Geometry check sheet. Reference: the model listing, model coordinates, mm. Coordinates: 2 decimals unless noted, no trailing zeros. Write each loop counter-clockwise with the first axis right and the second up, starting at its lowest first coordinate (ties: lowest second). Pieces come first, ordered by that corner, then holes. Notation, with made-up numbers: (-19, -24.75) -> (6, -24.75) arc R25 cw to (6, -7.75) -> close; hole circle Ø9 at (-29.75, 54). An arc over 180 degrees is marked (long way). One line per question, with ' | ' between items.
```python
from build123d import *

# Parameters (mm, degrees)
BOSS_EXTRUDE1_DEPTH = 450
SKETCH2_R           = 3
CUT_EXTRUDE1_DEPTH  = 4.5
SKETCH3_R           = 1.75
CUT_EXTRUDE2_DEPTH  = 451.09610085
LPATTERN1_COUNT     = 6
LPATTERN1_PITCH     = 80


with BuildPart() as part:
    # Sketch1 → Boss-Extrude1 (new body)
    with BuildSketch(Plane.XY):
        with BuildLine():
            Line((6.624531067, 2.444), (6.139791576, 2.444))
            ThreePointArc((6.139791576, 2.444), (5.3, 1.894), (6.139791576, 1.344))
            Line((6.139791576, 1.344), (6.624531067, 1.344))
            ThreePointArc((6.624531067, 1.344), (6.975900024, 0.857004226), (7.5, 0.563841739))
            Line((7.5, 0.563841739), (7.5, -4.2))
            Line((7.5, -4.2), (6.7, -5))
            Line((6.7, -5), (-6.7, -5))
            Line((-6.7, -5), (-7.5, -4.2))
            Line((-7.5, -4.2), (-7.5, 0.563841739))
            ThreePointArc((-7.5, 0.563841739), (-6.975900024, 0.857004226), (-6.624531067, 1.344))
            Line((-6.624531067, 1.344), (-6.139791576, 1.344))
            ThreePointArc((-6.139791576, 1.344), (-5.3, 1.894), (-6.139791576, 2.444))
            Line((-6.139791576, 2.444), (-6.624531067, 2.444))
            ThreePointArc((-6.624531067, 2.444), (-6.975900024, 2.930995774), (-7.5, 3.224158261))
            Line((-7.5, 3.224158261), (-7.5, 4.2))
            Line((-7.5, 4.2), (-6.7, 5))
            Line((-6.7, 5), (6.7, 5))
            Line((6.7, 5), (7.5, 4.2))
            Line((7.5, 4.2), (7.5, 3.224158261))
            ThreePointArc((7.5, 3.224158261), (6.975900024, 2.930995774), (6.624531067, 2.444))
        make_face()
    extrude(amount=-BOSS_EXTRUDE1_DEPTH)

    # Sketch2 → Cut-Extrude1 (cut)
    with BuildSketch(Plane(origin=(0, 5, 0), x_dir=(1, 0, 0), z_dir=(0, 1, 0))):
        with Locations(Location((0, 25, 0), (0, 0, 270))):
            Circle(SKETCH2_R)
    cut_extrude1 = extrude(amount=-CUT_EXTRUDE1_DEPTH, mode=Mode.SUBTRACT)

    # Sketch3 → Cut-Extrude2 (cut, through all)
    with BuildSketch(Plane(origin=(0, 0.5, 0), x_dir=(1, 0, 0), z_dir=(0, 1, 0))):
        with Locations(Location((0, 25, 0), (0, 0, 270))):
            Circle(SKETCH3_R)
    cut_extrude2 = extrude(amount=-CUT_EXTRUDE2_DEPTH, mode=Mode.SUBTRACT)

    # LPattern1: Cut-Extrude1, Cut-Extrude2 ×6
    with Locations(*[(0, 0, -i * LPATTERN1_PITCH) for i in range(1, LPATTERN1_COUNT)]):
        add(cut_extrude1, mode=Mode.SUBTRACT)
        add(cut_extrude2, mode=Mode.SUBTRACT)


solid = part.part
```
(1) Depth check by flat-ended pin: P1, Ø1, axis at y = 2, z = -352, coming from the -X side; P2, Ø4, axis at x = 0, z = -25, coming from the +Y side. Enter the tip coordinate at first touch or a pass-through.
Answers below:
P1: stops at x = -6.65 | P2: stops at y = 0.5
(2) Cross-section at A-A (z = -373.5). Record the cut outline in (x, y), plus the area to 3 significant figures.
Answers below:
outline: (-7.5, -4.2) -> (-6.7, -5) -> (6.7, -5) -> (7.5, -4.2) -> (7.5, 0.56) arc R1.39 cw to (6.62, 1.34) -> (6.14, 1.34) arc R0.6 cw (long way) to (6.14, 2.44) -> (6.62, 2.44) arc R1.39 cw to (7.5, 3.22) -> (7.5, 4.2) -> (6.7, 5) -> (-6.7, 5) -> (-7.5, 4.2) -> (-7.5, 3.22) arc R1.39 cw to (-6.62, 2.44) -> (-6.14, 2.44) arc R0.6 cw (long way) to (-6.14, 1.34) -> (-6.62, 1.34) arc R1.39 cw to (-7.5, 0.56) -> close | area: 142 mm²
(3) Material ranges on line 1 (X direction, y = 2.55, z = -105); line 2 (Y direction, x = 6, z = -237.5); line 3 (X direction, y = 1.7, z = -345), recorded low to high.
Answers below:
line 1: x = -6.68 to -3, 3 to 6.68 | line 2: y = -5 to 1.3, 2.49 to 5 | line 3: x = -5.33 to -3, 3 to 5.33
